```python
from build123d import *

# Parameters (mm, degrees)
F1_DEPTH      = 22.6695
F1_DEPTH_BACK = 22.6695
F3_DEPTH      = 25.4
F5_DEPTH      = 25.4
F7_DEPTH      = 25.4
F8_R          = 0.762


with BuildPart() as f1:
    # F0 (on Front) → F1 (new body, two sides)
    with BuildSketch(Plane.XZ) as f1_sk:
        Polygon((-17.78, 3.556), (-17.78, 0), (0, 0), (0, 26.67), (-4.064, 26.67), (-4.064, 3.556), align=None)
    extrude(amount=F1_DEPTH)
    extrude(f1_sk.sketch, amount=-F1_DEPTH_BACK)

    # F2 (on face) → F3 (cut)
    with BuildSketch(Plane.YZ):
        with BuildLine():
            Line((21.59, 3.556), (22.6695, 3.556))
            Line((22.6695, 3.556), (22.6695, 27.94))
            Line((22.6695, 27.94), (0, 27.94))
            Line((0, 27.94), (-22.6695, 27.94))
            Line((-22.6695, 27.94), (-22.6695, 3.556))
            Line((-22.6695, 3.556), (-21.59, 3.556))
            Line((-21.59, 3.556), (-21.59, 12.7))
            ThreePointArc((-21.59, 12.7), (-21.3970584633, 14.9053318564), (-20.824096284, 17.0436558202))
            Line((-20.824096284, 17.0436558202), (-18.5369777572, 23.3274623281))
            ThreePointArc((-18.5369777572, 23.3274623281), (-16.6771075403, 25.751292385), (-13.7633392436, 26.67))
            Line((-13.7633392436, 26.67), (-7.3148526832, 26.67))
            ThreePointArc((-7.3148526832, 26.67), (-3.7438138302, 25.2030432478), (-2.2352, 21.6494021693))
            Line((-2.2352, 21.6494021693), (-2.0953567318, 9.6909966051))
            ThreePointArc((-2.0953567318, 9.6909966051), (-1.4730535269, 8.2251196603), (0, 7.62))
            ThreePointArc((0, 7.62), (1.4730535269, 8.2251196603), (2.0953567318, 9.6909966051))
            Line((2.0953567318, 9.6909966051), (2.2352, 21.6494021693))
            ThreePointArc((2.2352, 21.6494021693), (3.7438138302, 25.2030432478), (7.3148526832, 26.67))
            Line((7.3148526832, 26.67), (13.7633392436, 26.67))
            ThreePointArc((13.7633392436, 26.67), (16.6771075403, 25.751292385), (18.5369777572, 23.3274623281))
            Line((18.5369777572, 23.3274623281), (20.824096284, 17.0436558202))
            ThreePointArc((20.824096284, 17.0436558202), (21.3970584633, 14.9053318564), (21.59, 12.7))
            Line((21.59, 12.7), (21.59, 3.556))
        make_face()
    extrude(amount=-F3_DEPTH, mode=Mode.SUBTRACT)

    # F4 (on face) → F5 (cut)
    with BuildSketch(Plane.XY.offset(3.556)):
        Polygon((0, 22.6695), (-2.1336, 22.6695), (-2.1336, 20.5486), (-0.9652, 20.5486), (-0.9652, 18.796), (0, 18.796), align=None)
        Polygon((-2.1336, -20.5486), (-2.1336, -22.6695), (0, -22.6695), (0, -18.796), (-0.9652, -18.796), (-0.9652, -20.5486), align=None)
    extrude(amount=F5_DEPTH, mode=Mode.SUBTRACT)

    # F6 (on face) → F7 (cut)
    with BuildSketch(Plane.XY.offset(3.556)):
        with BuildLine():
            ThreePointArc((-16.3926058311, 20.5171362549), (-8.2666528236, 22.1291096803), (0, 22.6695))
            Line((0, 22.6695), (0, 25.4))
            Line((0, 25.4), (-25.4, 25.4))
            Line((-25.4, 25.4), (-25.4, -25.4))
            Line((-25.4, -25.4), (0, -25.4))
            Line((0, -25.4), (0, -22.6695))
            ThreePointArc((0, -22.6695), (-8.2666528236, -22.1291096803), (-16.3926058311, -20.5171362549))
            ThreePointArc((-16.3926058311, -20.5171362549), (-17.78, 0), (-16.3926058311, 20.5171362549))
        make_face()
    extrude(amount=-F7_DEPTH, mode=Mode.SUBTRACT)

    # F8
    f8_edges = [f1.edges().sort_by_distance(p)[0] for p in [
        (-8.266653, -22.12911, 0),
        (-17.78, 0, 0),
        (-8.266653, 22.12911, 0),
        (-16.392606, -20.517136, 1.778),
        (-16.392606, 20.517136, 1.778),
        (-4.064, 21.59, 8.128),
        (0, 0, 7.62),
    ]]
    fillet(f8_edges, radius=F8_R)


solid = f1.part
```
Source: CAD feature listing. Evaluate the final solid. Frame: model axes, mm. A direction names the side the tool comes from. Round coordinates to 2 decimals unless told otherwise and drop trailing zeros. Loops run counter-clockwise (first coordinate to the right, second up) from the corner with the lowest first, then second, coordinate; pieces in that order, holes last. Notation, with made-up numbers: M 29,60.5 L 42,60.5 A27 ccw 42,79.5 Z; hole C 19,48.5 d5. An arc over 180 degrees is marked long. Use a Markdown table: item, result. Add a question column.
1. Reachability of faces 1 (the cylindrical face through (-2.01, -3.78, 25.24)), 2 (the flat face through (-2.134, -21, 11)), 3 (the flat face through (-3, 21.59, 8)), 4 (the flat face through (-3, -21.59, 8)) from +Z, -Z, +X, -X, +Y, -Y: full face, straight path, thin tool, end or side. Return the list, or none.
2. Mould query, pull axis Y, two halves, no side actions, for faces 5 (the cylindrical face through (-0.217, 2.395, 15.751)), 6 (the cylindrical face through (-2.014, 16.641, 25.776)), 7 (the flat face through (-0.5, -18.796, 13)). Classes: pulls with the +Y half, pulls with the -Y half, needs draft (parallel to the pull), parting line crosses it, or undercut.
3. Line query: line 1 (Z direction, x = -13, y = -19.5); line 2 (X direction, y = -17.5, z = 18.75); line 3 (Y direction, x = -1, z = 8.25). Output: solid intervals per line, ascending.
4. Contact query for flat-ended pins moving along their axis: P1, Ø8, axis at y = 8.5, z = 9.5, coming from the -X side; P2, Ø1.3, axis at x = -2.5, z = 10.5, coming from the -Y side; P3, Ø4, axis at x = -5.5, z = 16.5, coming from the +Y side. Output: stop coordinate, or through.
5. Section query A-A on z = 5.75. Return the cut outline in (x, y).
Reported:
| question | item | result |
|---|---|---|
| 1 | face 1 | +Z, +X, -X |
| 1 | face 2 | +Z, +X, -Y |
| 1 | face 3 | +Z, +X, -X, +Y |
| 1 | face 4 | +Z, +X, -X, -Y |
| 2 | face 5 | undercut |
| 2 | face 6 | pulls with the +Y half |
| 2 | face 7 | pulls with the -Y half |
| 3 | line 1 | z = 0 to 3.56 |
| 3 | line 2 | x = -4.06 to 0 |
| 3 | line 3 | y = -20.55 to -1.5, 1.5 to 20.55 |
| 4 | P1 | stops at x = -4.06 |
| 4 | P2 | stops at y = -21.59 |
| 4 | P3 | stops at y = 21.13 |
| 5 | outline | M -4.06,-20.83 A0.76 ccw -3.3,-21.59 L -2.13,-21.59 L -2.13,-20.55 L -0.97,-20.55 L -0.97,-18.8 L 0,-18.8 L 0,18.8 L -0.97,18.8 L -0.97,20.55 L -2.13,20.55 L -2.13,21.59 L -3.3,21.59 A0.76 ccw -4.06,20.83 Z |
